Autodesk Inventor part; units mm, degrees
ref_plane "YZ Plane" through (0, 0, 0) normal (1, 0, 0) x (0, 1, 0)
ref_plane "XZ Plane" through (0, 0, 0) normal (0, 1, 0) x (-1, 0, 0)
ref_plane "XY Plane" through (0, 0, 0) normal (0, 0, 1) x (1, 0, 0)
sketch "Sketch1" plane through (0, 0, 0) normal (0, 0, 1) x (1, 0, 0)
  line L0 (447.8771, 77.149) -> (316.286, 87.8713)
  line L1 (314.6655, 88.2204) -> (190.8775, 132.4412)
  line L2 (189.4026, 133.1978) -> (82.2199, 207.2992)
  line L3 (0, 202.0759) -> (0, 6.35)
  circle A0 centre (440.5162, 61.8212) radius 2.413
  circle A1 centre (320.4926, 71.6009) radius 2.413
  line L4 (448.1345, 77.128) -> (443.7313, 23.0895) construction
  line L5 (315.4528, 87.9391) -> (312.3268, 49.5751) construction
  line L6 (315.4528, 87.9391) -> (300.5748, 46.291) construction
  circle A2 centre (190.7297, 115.6365) radius 2.413
  circle A3 centre (304.1324, 75.1256) radius 2.413
  line L7 (190.0903, 132.7224) -> (175.3821, 91.5497) construction
  line L8 (190.0903, 132.7224) -> (160.9674, 90.5981) construction
  circle A4 centre (175.8392, 123.2754) radius 2.413
  circle A5 centre (76.7856, 191.7567) radius 2.413
  line L9 (80.5901, 208.4259) -> (54.0448, 170.0299) construction
  line L10 (69.85, 208.4259) -> (76.2, 208.4259)
  line L11 (76.2, 202.0759) -> (76.2, 208.4259) construction
  line L12 (448.3928, 77.128) -> (454.4845, 77.128)
  line L13 (12.7, 208.4259) -> (6.35, 208.4259)
  line L14 (78.6088, 208.4259) -> (63.5, 208.4259)
  line L15 (12.7, 208.4259) -> (63.5, 208.4259)
  line L16 (12.7, 202.0759) -> (31.75, 202.0759)
  line L17 (31.75, 202.0759) -> (31.75, 195.7259)
  line L18 (31.75, 195.7259) -> (12.7, 195.7259)
  line L19 (12.7, 195.7259) -> (12.7, 202.0759)
  line L20 (44.45, 202.0759) -> (63.5, 202.0759)
  line L21 (63.5, 202.0759) -> (63.5, 195.7259)
  line L22 (63.5, 195.7259) -> (44.45, 195.7259)
  line L23 (44.45, 195.7259) -> (44.45, 202.0759)
  line L24 (63.5, 195.7259) -> (71.8099, 195.7259) construction
  line L25 (71.8099, 195.7259) -> (71.8099, 208.4259) construction
  line L26 (12.7, 6.35) -> (31.75, 6.35)
  line L27 (31.75, 6.35) -> (31.75, 12.7)
  line L28 (31.75, 12.7) -> (12.7, 12.7)
  line L29 (12.7, 12.7) -> (12.7, 6.35)
  line L30 (69.85, 12.7) -> (88.9, 12.7)
  line L31 (88.9, 12.7) -> (88.9, 6.35)
  line L32 (88.9, 6.35) -> (69.85, 6.35)
  line L33 (69.85, 6.35) -> (69.85, 12.7)
  line L34 (127, 12.7) -> (146.05, 12.7)
  line L35 (146.05, 12.7) -> (146.05, 6.35)
  line L36 (146.05, 6.35) -> (127, 6.35)
  line L37 (127, 6.35) -> (127, 12.7)
  line L38 (184.15, 12.7) -> (203.2, 12.7)
  line L39 (203.2, 12.7) -> (203.2, 6.35)
  line L40 (203.2, 6.35) -> (184.15, 6.35)
  line L41 (184.15, 6.35) -> (184.15, 12.7)
  line L42 (241.3, 12.7) -> (260.35, 12.7)
  line L43 (260.35, 12.7) -> (260.35, 6.35)
  line L44 (260.35, 6.35) -> (241.3, 6.35)
  line L45 (241.3, 6.35) -> (241.3, 12.7)
  line L46 (298.45, 12.7) -> (317.5, 12.7)
  line L47 (317.5, 12.7) -> (317.5, 6.35)
  line L48 (317.5, 6.35) -> (298.45, 6.35)
  line L49 (298.45, 6.35) -> (298.45, 12.7)
  line L50 (355.6, 12.7) -> (374.65, 12.7)
  line L51 (374.65, 12.7) -> (374.65, 6.35)
  line L52 (374.65, 6.35) -> (355.6, 6.35)
  line L53 (355.6, 6.35) -> (355.6, 12.7)
  line L54 (412.75, 12.7) -> (431.8, 12.7)
  line L55 (431.8, 12.7) -> (431.8, 6.35)
  line L56 (431.8, 6.35) -> (412.75, 6.35)
  line L57 (412.75, 6.35) -> (412.75, 12.7)
  line L58 (460.8345, 70.778) -> (460.8345, 6.35)
  line L59 (454.4845, 0) -> (454.4845, 0)
  line L60 (448.1345, 12.7) -> (454.4845, 12.7)
  line L61 (454.4845, 12.7) -> (454.4845, 31.75)
  line L62 (454.4845, 31.75) -> (448.1345, 31.75)
  line L63 (448.1345, 31.75) -> (448.1345, 12.7)
  line L64 (448.1345, 51.728) -> (454.4845, 51.728)
  line L65 (454.4845, 51.728) -> (454.4845, 70.778)
  line L66 (454.4845, 70.778) -> (448.1345, 70.778)
  line L67 (448.1345, 70.778) -> (448.1345, 51.728)
  line L68 (6.35, 189.3759) -> (12.7, 189.3759)
  line L69 (12.7, 189.3759) -> (12.7, 170.3259)
  line L70 (12.7, 170.3259) -> (6.35, 170.3259)
  line L71 (6.35, 170.3259) -> (6.35, 189.3759)
  line L72 (6.35, 139.8459) -> (12.7, 139.8459)
  line L73 (12.7, 139.8459) -> (12.7, 120.7959)
  line L74 (12.7, 120.7959) -> (6.35, 120.7959)
  line L75 (6.35, 120.7959) -> (6.35, 139.8459)
  line L76 (6.35, 90.3159) -> (12.7, 90.3159)
  line L77 (12.7, 90.3159) -> (12.7, 71.2659)
  line L78 (12.7, 71.2659) -> (6.35, 71.2659)
  line L79 (6.35, 71.2659) -> (6.35, 90.3159)
  line L80 (6.35, 40.7859) -> (12.7, 40.7859)
  line L81 (12.7, 40.7859) -> (12.7, 21.7359)
  line L82 (12.7, 21.7359) -> (6.35, 21.7359)
  line L83 (6.35, 21.7359) -> (6.35, 40.7859)
  arc A6 (6.35, 208.4259) -> (0, 202.0759) centre (6.35, 202.0759) ccw
  arc A7 (82.2199, 207.2992) -> (78.6088, 208.4259) centre (78.6088, 202.0759) ccw
  arc A8 (189.4026, 133.1978) -> (190.8775, 132.4412) centre (193.0137, 138.4211) ccw
  arc A9 (314.6655, 88.2204) -> (316.286, 87.8713) centre (316.8017, 94.2003) ccw
  arc A10 (447.8771, 77.149) -> (448.3928, 77.128) centre (448.3928, 83.478) ccw
  arc A11 (460.8345, 70.778) -> (454.4845, 77.128) centre (454.4845, 70.778) ccw
  arc A12 (454.4845, 0) -> (460.8345, 6.35) centre (454.4845, 6.35) ccw
  arc A13 (0, 6.35) -> (6.35, 0) centre (6.35, 6.35) ccw
  line L84 (6.35, 0) -> (454.4845, 0)
  point P0 (0, 0)
  point P1 (0, 0)
  point P2 (460.8345, 77.128)
  dimension "d3" = 4.826
  dimension "d4" = 4.826
  dimension "d5" = 15.875
  dimension "d6" = 15.875
  dimension "d7" = 120.4214
  dimension "d8" = 90
  dimension "d9" = 6.35
  dimension "d11" = 90
  dimension "d12" = 90
  dimension "d13" = 165
  dimension "d14" = 6.35
  dimension "d16" = 4.826
  dimension "d17" = 4.826
  dimension "d18" = 6.35
  dimension "d19" = 15.875
  dimension "d20" = 15.875
  dimension "d21" = 120.4214
  dimension "d22" = 165
  dimension "d23" = 90
  dimension "d24" = 90
  dimension "d25" = 6.35
  dimension "d26" = 4.826
  dimension "d27" = 4.826
  dimension "d28" = 6.35
  dimension "d29" = 15.875
  dimension "d30" = 15.875
  dimension "d31" = 120.4214
  dimension "d32" = 90
  dimension "d33" = 6.35
  dimension "d38" = 6.35
  dimension "d39" = 12.7
  dimension "d41" = 76.2
  dimension "d76" = 19.05
  dimension "d77" = 6.35
  dimension "d78" = 19.05
  dimension "d79" = 6.35
  dimension "d80" = 12.7
  dimension "d81" = 12.7
  dimension "d82" = 6.35
  dimension "d83" = 6.35
  dimension "d84" = 71.8099
  dimension "d86" = 6.35
  dimension "d87" = 19.05
  dimension "d88" = 6.35
  dimension "d89" = 19.05
  dimension "d91" = 6.35
  dimension "d92" = 6.35
  dimension "d93" = 6.35
  dimension "d94" = 6.35
  dimension "d97" = 19.05
  dimension "d98" = 19.05
  dimension "d99" = 19.05
  dimension "d100" = 19.05
  dimension "d102" = 12.7
  dimension "d106" = 38.1
  dimension "d107" = 38.1
  dimension "d109" = 38.1
  dimension "d112" = 38.1
  dimension "d113" = 38.1
  dimension "d115" = 19.05
  dimension "d116" = 6.35
  dimension "d117" = 38.1
  dimension "d119" = 38.1
  dimension "d120" = 6.35
extrude "Extrusion2" add sketch "Sketch1" along normal blind 6.35
equation "\"d4\" = d3"
equation "\"d5\" = d6"
equation "\"d14\" = d9"
equation "\"d16\" = d3"
equation "\"d17\" = d3"
equation "\"d18\" = d9"
equation "\"d19\" = d6"
equation "\"d20\" = d6"
equation "\"d21\" = d7"
equation "\"d22\" = d13"
equation "\"d25\" = d9"
equation "\"d26\" = d3"
equation "\"d27\" = d3"
equation "\"d28\" = d9"
equation "\"d29\" = d6"
equation "\"d30\" = d6"
equation "\"d31\" = d7"
equation "\"d33\" = d9"
equation "\"d78\" = d76"
equation "\"d81\" = d80"
equation "\"d83\" = d82"
equation "\"d86\" = d77"
equation "\"d87\" = d76"
equation "\"d88\" = d86"
equation "\"d89\" = d87"
equation "\"d91\" = d86"
equation "\"d92\" = d86"
equation "\"d93\" = d86"
equation "\"d94\" = d93"
properties part number "9U Cheek V3"
Geometry: final body of the model. Coordinates: model frame, mm. Coordinates: 2 decimals unless noted, no trailing zeros. Order: outer loops, then holes, each group sorted by start corner. A loop starts at its lowest first (then second) coordinate and runs counter-clockwise, first axis right, second up. Notation, with made-up numbers: (47, 34.25) - (59, 34.25) arc R32 ccw to (59, 69.25) - close; hole circle Ø10 at (73, 44). An arc over 180 degrees is marked (long way). Return JSON: item names as keys, results as strings. Group by question number.
1. Cut plane B-B (y = 99). Output: boundary loops of the cut face in (x, z).
2. Cut plane C-C (z = 2.75). Count the separate pieces of the cut face and the enclosed holes in it, plus the area to 3 significant figures.
3. Material intervals for line 1 along Y through (x, z) = (20, 4.5); line 2 along Y through (x, z) = (422, 6); line 3 along X through (y, z) = (71, 1.75), sorted ascending. Write a range as [from, to].
4. Cut plane A-A (x = 365.5). Output: boundary loops of the cut face in (y, z).
5. Pin query (flat end, axial travel): pin 1 (1.9 mm diameter, centred on x = 197.5, z = 1.5, fed in from +Y); pin 2 (4.5 mm diameter, centred on x = 76.79, y = 191.76, fed in from -Z); pin 3 (3 mm diameter, centred on x = 309.5, z = 4, fed in from +Y). Return the tip coordinate at first contact, or that it passes through.
Resolved:
{
 "1": {"outline": "(0, 0) - (284.49, 0) - (284.49, 6.35) - (0, 6.35) - close"},
 "2": {"separate pieces": "1", "enclosed holes": "22", "area": "59,200 mm²"},
 "3": {"line 1": "y = [0, 6.35], [12.7, 195.73], [202.08, 208.43]", "line 2": "y = [0, 6.35], [12.7, 79.26]", "line 3": "x = [0, 318.16], [322.83, 460.83]"},
 "4": {"outline": "(0, 0) - (6.35, 0) - (6.35, 6.35) - (0, 6.35) - close; (12.7, 0) - (83.86, 0) - (83.86, 6.35) - (12.7, 6.35) - close"},
 "5": {"pin 1": "stops at y = 130.41", "pin 2": "passes through", "pin 3": "stops at y = 90.6"}
}
